Verification items for the finished model (mm, model axes). A direction names the side the tool comes from. Round coordinates to 2 decimals unless told otherwise and drop trailing zeros. Order: outer loops, then holes, each group sorted by start corner. A loop starts at its lowest first (then second) coordinate and runs counter-clockwise, first axis right, second up. Notation, with made-up numbers: (-25.75, -26.5) -> (-6.75, -26.5) arc R9 ccw to (-6.75, -14.5) -> close; hole circle Ø6 at (37.25, 67.25). An arc over 180 degrees is marked (long way). Answer in a Markdown table with one row per item. Add a question column.
```python
from build123d import *

# Parameters (mm, degrees)
F0_R     = 12.7
F0_R_2   = 10.922
F1_DEPTH = 19.05
F3_R     = 9.779
F3_R_2   = 8.382
F4_DEPTH = 7.62
F5_R     = 12.7
F5_R_2   = 9.906
F6_DEPTH = 19.05


with BuildPart() as f1:
    # F0 (on Top) → F1 (new body)
    with BuildSketch(Plane.XY):
        with Locations((-25.4, 25.4)):
            Circle(F0_R)
        with Locations((-25.4, 25.4)):
            Circle(F0_R_2, mode=Mode.SUBTRACT)
    extrude(amount=F1_DEPTH)



with BuildPart() as f4:
    # F3 (on offset) → F4 (new body)
    with BuildSketch(Plane.XZ.offset(-12.7)):
        with Locations((-25.4, 47.3280113715)):
            Circle(F3_R)
        with Locations((-25.4, 47.3280113715)):
            Circle(F3_R_2, mode=Mode.SUBTRACT)
    extrude(amount=-F4_DEPTH)


with BuildPart() as f1_1:
    add(f1.part)

    add(f4.part)  # F6 merges F4
    # F5 (on face) → F6 (join)
    with BuildSketch(Plane.XY.offset(19.05)):
        with Locations((-25.4, 25.4)):
            Circle(F5_R)
        with Locations((-25.4, 25.4)):
            Circle(F5_R_2, mode=Mode.SUBTRACT)
    extrude(amount=F6_DEPTH)


solid = f1_1.part
```
1) Tool access check on faces 4 (the face through (-15.31, 21.22, 9.39)), 5 (the face through (-18, 12.7, 52)). Record the directions out of +Z, -Z, +X, -X, +Y, -Y that give a thin tool (end or side, any length) a straight path to the whole face; none if there is none.
2) Thickness scan on L1, parallel to Y at x = -25.4, z = 9.25; L2, parallel to Z at x = -25.4, y = 16.75; L3, parallel to Y at x = -33, z = 13. Record the ranges inside material, lowest first. Write a range as [from, to].
3) Cross-section at D-D, the plane z = 6.5. Record the boundary of the cut face in (x, y).
4) Cross-section at A-A, the plane y = 19. Record the boundary of the cut face in (x, z), and give its area (3 significant figures).
5) Draft check along X on faces 1 (the face through (-20.6, 16.55, 19.05)), 2 (the face through (-22, 36, 0)), 3 (the face through (-18.573, 36.109, 18.783)). Enter one of: +X half, -X half, draft (parallel to the pull), parting line (faces both ways), or undercut.
6) Cross-section at B-B, the plane x = -23. Record the boundary of the cut face in (y, z), and give its area (3 significant figures).
7) Depth check by flat-ended pin: P1, Ø6.5, axis at x = -27.5, y = 25, coming from the -Z side; P2, Ø6, axis at y = 30, z = 27, coming from the +X side; P3, Ø6, axis at x = -20.5, y = 19.5, coming from the +Z side; P4, Ø1, axis at x = -20.5, y = 20, coming from the +Z side. Enter the tip coordinate at first touch or a pass-through.
8) Cross-section at C-C, the plane y = 25.4. Record the boundary of the cut face in (x, z), and give its area (3 significant figures).
Results below:
| question | item | result |
|---|---|---|
| 1 | face 4 | -Z |
| 1 | face 5 | +Z, -Z, +X, -X, -Y |
| 2 | L1 | [12.7, 14.48], [36.32, 38.1] |
| 2 | L2 | [37.55, 38.95], [55.71, 57.11] |
| 2 | L3 | [15.23, 17.56], [33.24, 35.57] |
| 3 | outline | circle Ø25.4 at (-25.4, 25.4); hole circle Ø21.84 at (-25.4, 25.4) |
| 4 | outline | (-36.37, 0) -> (-34.25, 0) -> (-34.25, 19.05) -> (-32.96, 19.05) -> (-32.96, 38.1) -> (-36.37, 38.1) -> close; circle Ø19.56 at (-25.4, 47.33); (-17.84, 19.05) -> (-16.55, 19.05) -> (-16.55, 0) -> (-14.43, 0) -> (-14.43, 38.1) -> (-17.84, 38.1) -> close; hole circle Ø16.76 at (-25.4, 47.33) |
| 4 | area | 290 mm² |
| 5 | face 1 | undercut |
| 5 | face 2 | draft |
| 5 | face 3 | parting line |
| 6 | outline | (12.7, 37.85) -> (12.93, 37.85) -> (12.93, 0) -> (14.74, 0) -> (14.74, 19.05) -> (15.79, 19.05) -> (15.79, 37.85) -> (20.32, 37.85) -> (20.32, 39.3) -> (12.7, 39.3) -> close; (12.7, 55.36) -> (20.32, 55.36) -> (20.32, 56.81) -> (12.7, 56.81) -> close; (35.01, 19.05) -> (36.06, 19.05) -> (36.06, 0) -> (37.87, 0) -> (37.87, 38.1) -> (35.01, 38.1) -> close |
| 6 | area | 200 mm² |
| 7 | P1 | through |
| 7 | P2 | x = -12.8 |
| 7 | P3 | z = 56.92 |
| 7 | P4 | z = 56.06 |
| 8 | outline | (-38.1, 0) -> (-36.32, 0) -> (-36.32, 19.05) -> (-35.31, 19.05) -> (-35.31, 38.1) -> (-38.1, 38.1) -> close; (-15.49, 19.05) -> (-14.48, 19.05) -> (-14.48, 0) -> (-12.7, 0) -> (-12.7, 38.1) -> (-15.49, 38.1) -> close |
| 8 | area | 174 mm² |
